Could you check a few things on this model? Use its own coordinates, in mm. A direction names the side the tool comes from. Round coordinates to 2 decimals unless told otherwise and drop trailing zeros. Loops run counter-clockwise (first coordinate to the right, second up) from the corner with the lowest first, then second, coordinate; pieces in that order, holes last. Notation, with made-up numbers: M 18.5,35.5 L 70.5,35.5 A7 ccw 70.5,48.5 Z; hole C -32.5,-35.75 d7. An arc over 180 degrees is marked long. Answer in a Markdown table with one row per item.
```python
from build123d import *

# Parameters (mm, degrees)
PRISM001_DEPTH             = 10
PRISM002_DEPTH             = 10
PRISM003_DEPTH             = 10
PRISM_DEPTH                = 10
CUBE001_W                  = 12
CUBE001_H                  = 16.5
CUBE001_DEPTH              = 10.85
CUBE_W                     = 143
CUBE_H                     = 84.23
CUBE_DEPTH                 = 1.6
DIFFERENCE_PLACEMENT_ANGLE = -90


with BuildPart() as prism001:
    # prism001 → prism001 (new body)
    with BuildSketch(Plane(origin=(139, 4, -1), x_dir=(1, 0, 0), z_dir=(0, 0, 1))):
        Polygon((2, 0), (1.902113, 0.618034), (1.618034, 1.175571), (1.175571, 1.618034), (0.618034, 1.902113), (0, 2), (-0.618034, 1.902113), (-1.175571, 1.618034), (-1.618034, 1.175571), (-1.902113, 0.618034), (-2, 0), (-1.902113, -0.618034), (-1.618034, -1.175571), (-1.175571, -1.618034), (-0.618034, -1.902113), (0, -2), (0.618034, -1.902113), (1.175571, -1.618034), (1.618034, -1.175571), (1.902113, -0.618034), align=None)
    extrude(amount=PRISM001_DEPTH)


with BuildPart() as prism002:
    # prism002 → prism002 (new body)
    with BuildSketch(Plane(origin=(4, 80.23, -1), x_dir=(1, 0, 0), z_dir=(0, 0, 1))):
        Polygon((2, 0), (1.902113, 0.618034), (1.618034, 1.175571), (1.175571, 1.618034), (0.618034, 1.902113), (0, 2), (-0.618034, 1.902113), (-1.175571, 1.618034), (-1.618034, 1.175571), (-1.902113, 0.618034), (-2, 0), (-1.902113, -0.618034), (-1.618034, -1.175571), (-1.175571, -1.618034), (-0.618034, -1.902113), (0, -2), (0.618034, -1.902113), (1.175571, -1.618034), (1.618034, -1.175571), (1.902113, -0.618034), align=None)
    extrude(amount=PRISM002_DEPTH)


with BuildPart() as prism003:
    # prism003 → prism003 (new body)
    with BuildSketch(Plane(origin=(139, 80.23, -1), x_dir=(1, 0, 0), z_dir=(0, 0, 1))):
        Polygon((2, 0), (1.902113, 0.618034), (1.618034, 1.175571), (1.175571, 1.618034), (0.618034, 1.902113), (0, 2), (-0.618034, 1.902113), (-1.175571, 1.618034), (-1.618034, 1.175571), (-1.902113, 0.618034), (-2, 0), (-1.902113, -0.618034), (-1.618034, -1.175571), (-1.175571, -1.618034), (-0.618034, -1.902113), (0, -2), (0.618034, -1.902113), (1.175571, -1.618034), (1.618034, -1.175571), (1.902113, -0.618034), align=None)
    extrude(amount=PRISM003_DEPTH)


with BuildPart() as group002:
    # prism → prism (new body)
    with BuildSketch(Plane(origin=(4, 4, -1), x_dir=(1, 0, 0), z_dir=(0, 0, 1))):
        Polygon((2, 0), (1.902113, 0.618034), (1.618034, 1.175571), (1.175571, 1.618034), (0.618034, 1.902113), (0, 2), (-0.618034, 1.902113), (-1.175571, 1.618034), (-1.618034, 1.175571), (-1.902113, 0.618034), (-2, 0), (-1.902113, -0.618034), (-1.618034, -1.175571), (-1.175571, -1.618034), (-0.618034, -1.902113), (0, -2), (0.618034, -1.902113), (1.175571, -1.618034), (1.618034, -1.175571), (1.902113, -0.618034), align=None)
    extrude(amount=PRISM_DEPTH)

    # Group002: union prism001, prism002, prism003
    add(prism001.part)
    add(prism002.part)
    add(prism003.part)


with BuildPart() as cube001:
    # cube001 → cube001 (new body)
    with BuildSketch(Plane(origin=(21.71, 0, 0), x_dir=(1, 0, 0), z_dir=(0, 0, 1))):
        with Locations((6, 8.25)):
            Rectangle(CUBE001_W, CUBE001_H)
    extrude(amount=CUBE001_DEPTH)


with BuildPart() as obj1:
    # cube → cube (new body)
    with BuildSketch(Plane.XY):
        with Locations((71.5, 42.115)):
            Rectangle(CUBE_W, CUBE_H)
    extrude(amount=CUBE_DEPTH)

    # Group001: union cube001
    add(cube001.part)

    # difference: cut Group002
    add(group002.part, mode=Mode.SUBTRACT)


with BuildPart() as obj1_1:
    # difference placement: moved
    add(obj1.part.moved(Location((0.5, 147, 4))).rotate(Axis((0.5, 147, 4), (0, 0, 1)), DIFFERENCE_PLACEMENT_ANGLE))


solid = obj1_1.part
```
1) I want a section at A-A, the plane x = 14. Please give me the cut outline in (y, z).
Computed:
| item | result |
|---|---|
| outline | M 4,4 L 147,4 L 147,5.6 L 125.29,5.6 L 125.29,14.85 L 113.29,14.85 L 113.29,5.6 L 4,5.6 Z |
2) Which directions (+Z, -Z, +X, -X, +Y, -Y) give clear straight access to the entire face, cutting with the end or side of a thin tool? Please do faces 1 (the face through (9, 113.29, 10)), 2 (the face through (9, 119, 14.85)), 3 (the face through (9, 125.29, 10)), 4 (the face through (17, 119, 10)).
Computed:
| item | result |
|---|---|
| face 1 | +Z, +X, -X, -Y |
| face 2 | +Z, +X, -X, +Y, -Y |
| face 3 | +Z, +X, -X, +Y |
| face 4 | +Z, +X, +Y, -Y |
3) I want a section at D-D, the plane x = 38. Please give me the cut outline in (y, z).
Computed:
| item | result |
|---|---|
| outline | M 4,4 L 147,4 L 147,5.6 L 4,5.6 Z |
4) I want a section at C-C, the plane z = 9.5. Please give me the cut outline in (x, y), plus the area to 3 significant figures.
Computed:
| item | result |
|---|---|
| outline | M 0.5,113.29 L 17,113.29 L 17,125.29 L 0.5,125.29 Z |
| area | 198 mm² |
5) Will these pins go through, and if not, where does the flat tip stop? P1, Ø4.5, axis at y = 120.5, z = 8.5, coming from the +X side; P2, Ø1, axis at x = 25.5, y = 68.5, coming from the +Z side; P3, Ø3, axis at x = 5.5, z = 8, coming from the +Y side.
Computed:
| item | result |
|---|---|
| P1 | stops at x = 17 |
| P2 | stops at z = 5.6 |
| P3 | stops at y = 125.29 |
6) I need wall thicknesses on line 1 (Y direction, x = 9.5, z = 13.25); line 2 (Y direction, x = 79.5, z = 5); line 3 (Z direction, x = 39, y = 100.5). Which ranges of each line are inside material? Lowest first, please.
Computed:
| item | result |
|---|---|
| line 1 | y = 113.29 to 125.29 |
| line 2 | y = 4 to 6.44, 9.56 to 141.44, 144.56 to 147 |
| line 3 | z = 4 to 5.6 |
7) I want a section at B-B, the plane y = 119.5. Please give me the cut outline in (x, z), plus the area to 3 significant figures.
Computed:
| item | result |
|---|---|
| outline | M 0.5,4 L 84.73,4 L 84.73,5.6 L 17,5.6 L 17,14.85 L 0.5,14.85 Z |
| area | 287 mm² |
